from build123d import *

# Parameters (mm, degrees)
FILLET2_R            = 1
CUT_EXTRUDE2_DEPTH   = 5
CUT_EXTRUDE2_DRAFT   = -30
MIRROR1_COPY_1_DEPTH = 5
MIRROR1_COPY_1_DRAFT = -30


with BuildPart() as part:
    # Sketch2 → Revolve1 (revolve)
    with BuildSketch(Plane(origin=(0, 0, 0), x_dir=(0, 0, -1), z_dir=(1, 0, 0)), mode=Mode.PRIVATE) as revolve1_sk:
        Polygon((-7, 16.5), (-7, 3), (0, 3), (0, 13.5), (-3, 13.5), (-3, 16.5), align=None)
        Polygon((0, 13.5), (0, 3), (7, 3), (7, 16.5), (3, 16.5), (3, 13.5), align=None)
    revolve(revolve1_sk.sketch.rotate(Axis((0, 0, 0), (0, 0, -1)), 90), axis=Axis((0, 0, 0), (0, 0, -1)))

    # Fillet2
    fillet2_edges = [part.edges().sort_by_distance(p)[0] for p in [
        (-16.5, 0, -3),
        (-16.5, 0, 3),
    ]]
    fillet(fillet2_edges, radius=FILLET2_R)


with BuildPart() as cut_extrude2_tool:
    # Sketch5 → Cut-Extrude2 (with draft: the straight prism first)
    with BuildSketch(Plane(origin=(0, 0, -7), x_dir=(-1, 0, 0), z_dir=(0, 0, -1))):
        Polygon((0, 9.237604307), (-8, 4.618802154), (-8, -4.618802154), (0, -9.237604307), (8, -4.618802154), (8, 4.618802154), align=None)
    extrude(amount=-CUT_EXTRUDE2_DEPTH)
    # Cut-Extrude2: the draft: its side faces are tilted about the plane it starts from
    cut_extrude2_sides = [cut_extrude2_tool.faces().sort_by_distance(p)[0] for p in [
        (4, 6.92820323, -4.5),
        (8, 0, -4.5),
        (4, -6.92820323, -4.5),
        (-4, -6.92820323, -4.5),
        (-8, 0, -4.5),
        (-4, 6.92820323, -4.5),
    ]]
    draft(cut_extrude2_sides, Plane(origin=(0, 0, -7), x_dir=(-1, 0, 0), z_dir=(0, 0, -1)), CUT_EXTRUDE2_DRAFT)


with BuildPart() as part_1:
    add(part.part)

    # Cut-Extrude2: cut by cut_extrude2_tool
    add(cut_extrude2_tool.part, mode=Mode.SUBTRACT)


with BuildPart() as mirror1_copy_1_tool:
    # Mirror1 copy 1 sketch → Mirror1 copy 1 (with draft: the straight prism first)
    with BuildSketch(Plane(origin=(0, 0, 7), x_dir=(-1, 0, 0), z_dir=(0, 0, 1))):
        Polygon((0, -9.237604307), (-8, -4.618802154), (-8, 4.618802154), (0, 9.237604307), (8, 4.618802154), (8, -4.618802154), align=None)
    extrude(amount=-MIRROR1_COPY_1_DEPTH)
    # Mirror1 copy 1: the draft: its side faces are tilted about the plane it starts from
    mirror1_copy_1_sides = [mirror1_copy_1_tool.faces().sort_by_distance(p)[0] for p in [
        (4, 6.92820323, 4.5),
        (8, 0, 4.5),
        (4, -6.92820323, 4.5),
        (-4, -6.92820323, 4.5),
        (-8, 0, 4.5),
        (-4, 6.92820323, 4.5),
    ]]
    draft(mirror1_copy_1_sides, Plane(origin=(0, 0, 7), x_dir=(-1, 0, 0), z_dir=(0, 0, 1)), MIRROR1_COPY_1_DRAFT)


with BuildPart() as part_2:
    add(part_1.part)

    # Mirror1 copy 1: cut by mirror1_copy_1_tool
    add(mirror1_copy_1_tool.part, mode=Mode.SUBTRACT)


solid = part_2.part
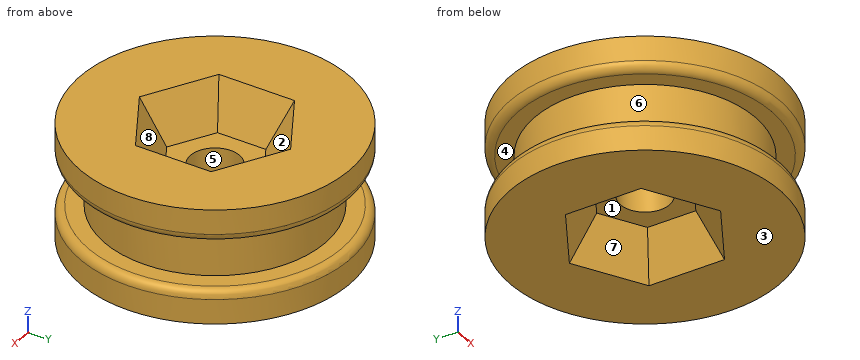
Build history of the part. All positions in model axes, mm. Face numbers are marked on the shaded views. A direction names the side the tool comes from. Coordinates: 2 decimals unless noted, no trailing zeros. Order: outer loops, then holes, each group sorted by start corner. A loop starts at its lowest first (then second) coordinate and runs counter-clockwise, first axis right, second up. Notation, with made-up numbers: (-13.75, 68.5) - (38.25, 68.5) arc R20 ccw to (38.25, 79.5) - close; hole circle Ø7 at (52, 87). An arc over 180 degrees is marked (long way). Write item = value, one per line. Start each with the question number.
1) Wall check: line 1 along Z through (x, y) = (1.5, 13.5); line 2 along Y through (x, z) = (0, 1); line 3 along Z through (x, y) = (8.5, 14). Give the ranges that are in metal, low to high. Write a range as from..to.
2) Saw through at C-C on z = 0.25. Write the cut outline in (x, y), then the cut area to 3 significant figures.
3) Saw through at B-B on z = -4.75. Write the cut outline in (x, y), then the cut area to 3 significant figures.
4) Two-plate mould, pull along Z, no slides. Class the marked faces 5, 6, 7 and 8: pulls with the +Z half, pulls with the -Z half, needs draft (parallel to the pull), parting line crosses it, or undercut.
5) Saw through at A-A on y = 0. Write the cut outline in (x, z).
6) 3-axis set-ups, long thin cutter, end or side, ignore diameter. For the marked faces 1, 2, 3 and 4: which of +Z, -Z, +X, -X, +Y, -Y reach the whole face in a straight line?
7) Flat gauge pins, fed straight in: pin 1 Ø9.5 at (x, y) = (0, 0) entering from +Z; pin 2 Ø5 at (x, y) = (-2, -1) entering from -Z; pin 3 Ø5 at (x, z) = (-11.5, 3) entering from -Y. Where does each tip first touch, or does it go through?
From the geometry:
q1.line_1 = -7..-3, 3..7
q1.line_2 = -13.5..-3, 3..13.5
q1.line_3 = -7..-3.52, 3.52..7
q2.outline = circle Ø27 at (0, 0); hole circle Ø6 at (0, 0)
q2.area = 544 mm^2
q3.outline = circle Ø33 at (0, 0); hole (-6.7, -3.87) - (0, -7.74) - (6.7, -3.87) - (6.7, 3.87) - (0, 7.74) - (-6.7, 3.87) - close
q3.area = 700 mm^2
q4.face_5 = needs draft
q4.face_6 = undercut
q4.face_7 = pulls with the -Z half
q4.face_8 = pulls with the +Z half
q5.outline = (-16.5, -7) - (-8, -7) - (-5.11, -2) - (-3, -2) - (-3, 2) - (-5.11, 2) - (-8, 7) - (-16.5, 7) - (-16.5, 4) arc R1 ccw to (-15.5, 3) - (-13.5, 3) - (-13.5, -3) - (-15.5, -3) arc R1 ccw to (-16.5, -4) - close; (3, -2) - (5.11, -2) - (8, -7) - (16.5, -7) - (16.5, -4) arc R1 ccw to (15.5, -3) - (13.5, -3) - (13.5, 3) - (15.5, 3) arc R1 ccw to (16.5, 4) - (16.5, 7) - (8, 7) - (5.11, 2) - (3, 2) - close
q6.face_1 = -Z
q6.face_2 = +Z
q6.face_3 = -Z, +X, -X, +Y, -Y
q6.face_4 = none
q7.pin_1 = 2
q7.pin_2 = -2
q7.pin_3 = -13.72
